Can you work these out from the drawing? Everything is in mm from the part's minimum corner. A direction names the side the tool comes from. Coordinates: 2 decimals unless noted, no trailing zeros. Loops run counter-clockwise (first coordinate to the right, second up) from the corner with the lowest first, then second, coordinate; pieces in that order, holes last. Notation, with made-up numbers: M 66.5,-30.75 L 75.5,-30.75 A20 cw 75.5,-14.75 Z; hole C 5.25,51 d4. An arc over 180 degrees is marked long. Use CSV: the item, a comma, the result in double quotes. Start each with the question number.
Q1. If we section it at B-B (y = 16.75): Please give me the cut outline in (x, z), and give its area (3 significant figures).
Q2. Which directions (+Z, -Z, +X, -X, +Y, -Y) give clear straight access to the entire face, cutting with the end or side of a thin tool? Please do the marked faces 4, 5 and 6.
Q3. For pin 1 Ø5 at (x, y) = (29.5, 9) entering from -Z; pin 2 Ø2 at (x, z) = (35.5, 9) entering from +Y; pin 3 Ø2 at (x, y) = (11.5, 8.5) entering from +Z; pin 4 Ø2 at (y, z) = (15.5, 1.5) entering from +X, each with a flat end and sliding along its axis, tell me the tip position at first contact or that it passes through.
Q4. Please list where these lines run through material, in increasing order: probe 1 along Z at (x, y) = (17.11, 0.95); probe 2 along Y at (x, z) = (46, 2.95); probe 3 along X at (y, z) = (1.5, 4.5). Write a range as [from, to].
Q5. If we section it at A-A (x = 46): Please give me the cut outline in (y, z), and give its area (3 significant figures).
Q6. If we section it at C-C (z = 2.5): Please give me the cut outline in (x, y), and give its area (3 significant figures).
Q7. If we section it at D-D (y = 6.25): Please give me the cut outline in (x, z), and give its area (3 significant figures).
Q8. If we mould it in two halves opening along Y, with no side actions, what happens to the marked faces 1, 2 and 3? For each: +Y half, -Y half, draft (parallel to the pull), parting line (faces both ways), or undercut.
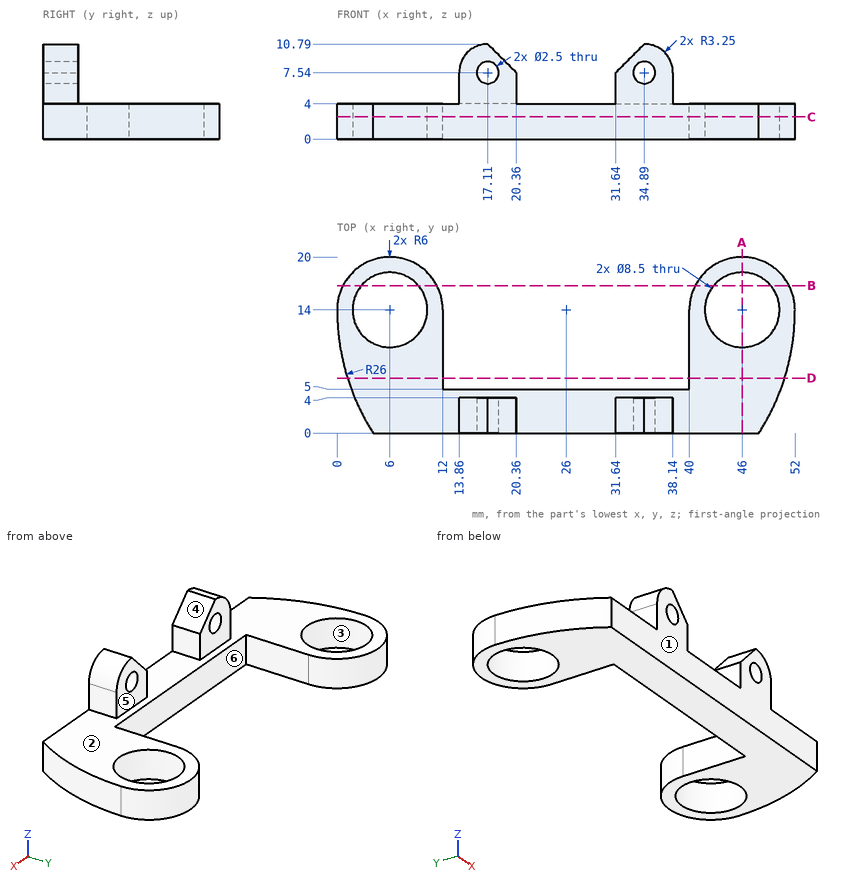
Results below:
1,outline,"M 0.67,0 L 2.76,0 L 2.76,4 L 0.67,4 Z; M 9.24,0 L 11.33,0 L 11.33,4 L 9.24,4 Z; M 40.67,0 L 42.76,0 L 42.76,4 L 40.67,4 Z; M 49.24,0 L 51.33,0 L 51.33,4 L 49.24,4 Z"
1,area,"33.5 mm^2"
2,face 4,"+Z, +Y, -Y"
2,face 5,"+Z, +X, -X, +Y"
2,face 6,"+Z, -Z, +Y"
3,pin 1,"through"
3,pin 2,"y = 4"
3,pin 3,"z = 4"
3,pin 4,"x = 51.98"
4,probe 1,"[0, 6.29], [8.79, 10.79]"
4,probe 2,"[0, 9.75], [18.25, 20]"
4,probe 3,"[13.86, 20.36], [31.64, 38.14]"
5,outline,"M 0,0 L 9.75,0 L 9.75,4 L 0,4 Z; M 18.25,0 L 20,0 L 20,4 L 18.25,4 Z"
5,area,"46.0 mm^2"
6,outline,"M 0,14 A26 ccw 4.09,0 L 47.91,0 A26 ccw 52,14 A6 ccw 40,14 L 40,5 L 12,5 L 12,14 A6 ccw Z; hole C 6,14 d8.5; hole C 46,14 d8.5"
6,area,"439 mm^2"
7,outline,"M 1.18,0 L 12,0 L 12,4 L 1.18,4 Z; M 40,0 L 50.82,0 L 50.82,4 L 40,4 Z"
7,area,"86.5 mm^2"
8,face 1,"-Y half"
8,face 2,"draft"
8,face 3,"undercut"
